Geometry check sheet. Reference: the model listing, model coordinates, mm. Face numbers are marked on the shaded views. Round coordinates to 2 decimals unless told otherwise and drop trailing zeros. Order: outer loops, then holes, each group sorted by start corner. A loop starts at its lowest first (then second) coordinate and runs counter-clockwise, first axis right, second up. Notation, with made-up numbers: (-20.75, -30.5) - (6.25, -30.5) arc R9 ccw to (6.25, -21.5) - close; hole circle Ø5 at (-12, 25.5). An arc over 180 degrees is marked (long way). Write each question's results on one line, items separated by ' | '.
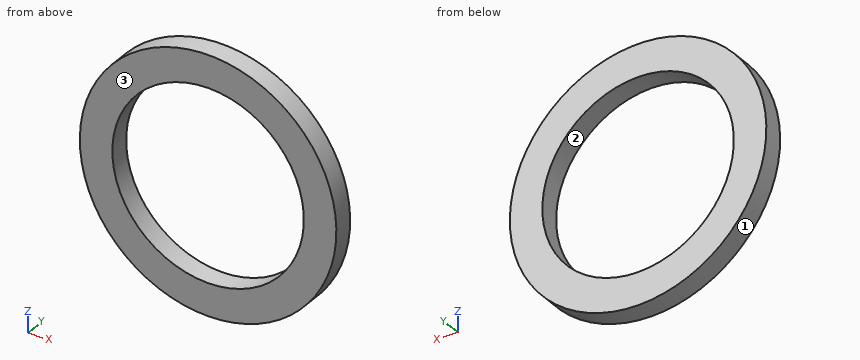
```python
from build123d import *

# Parameters (mm, degrees)
SKETCH1_R           = 19.05
BOSS_EXTRUDE1_DEPTH = 3.048
SKETCH2_R           = 14.224
CUT_EXTRUDE1_DEPTH  = 28.112641037


with BuildPart() as part:
    # Sketch1 → Boss-Extrude1 (new body)
    with BuildSketch(Plane(origin=(0, 0, 0), x_dir=(1, 0, 0), z_dir=(0, 1, 0))):
        with Locations(Location((0, 0, 0), (0, 0, 90))):
            Circle(SKETCH1_R)
    extrude(amount=BOSS_EXTRUDE1_DEPTH)

    # Sketch2 → Cut-Extrude1 (cut, through all)
    with BuildSketch(Plane(origin=(0, 3.048, 0), x_dir=(1, 0, 0), z_dir=(0, 1, 0))):
        with Locations(Location((0, 0, 0), (0, 0, 270))):
            Circle(SKETCH2_R)
    extrude(amount=-CUT_EXTRUDE1_DEPTH, mode=Mode.SUBTRACT)


solid = part.part
```
(1) Section check C-C (y = 0.95). Record the cut outline in (x, z).
Answers follow:
outline: circle Ø38.1 at (0, 0); hole circle Ø28.45 at (0, 0)
(2) Section check B-B (x = 0). Record the cut outline in (y, z), then the cut area to 3 significant figures.
Answers follow:
outline: (0, -19.05) - (3.05, -19.05) - (3.05, -14.22) - (0, -14.22) - close; (0, 14.22) - (3.05, 14.22) - (3.05, 19.05) - (0, 19.05) - close | area: 29.4 mm²
(3) Section check A-A (z = 0). Record the cut outline in (x, y), then the cut area to 3 significant figures.
Answers follow:
outline: (-19.05, 0) - (-14.22, 0) - (-14.22, 3.05) - (-19.05, 3.05) - close; (14.22, 0) - (19.05, 0) - (19.05, 3.05) - (14.22, 3.05) - close | area: 29.4 mm²
(4) Draft check along Z on the marked faces 1, 2 and 3. Enter one of: released by +Z, released by -Z, zero draft, split by the parting line, or undercut.
Answers follow:
face 1: split by the parting line | face 2: undercut | face 3: zero draft
(5) Material ranges on line 1 (X direction, y = 2.15, z = 0); line 2 (Z direction, x = -4, y = 2.05); line 3 (X direction, y = 0.75, z = -3), recorded low to high.
Answers follow:
line 1: -19.05 to -14.22, 14.22 to 19.05 | line 2: -18.63 to -13.65, 13.65 to 18.63 | line 3: -18.81 to -13.9, 13.9 to 18.81
(6) Depth check by flat-ended pin: pin 1 Ø1 at (x, y) = (-2.5, 2.5) entering from -Z. Enter the tip coordinate at first touch or a pass-through.
Answers follow:
pin 1: z = -18.94
